from build123d import *

# Parameters (mm, degrees)
F0_W     = 12.1070817113
F0_H     = 12.026887387
F1_DEPTH = 50.8
F2_R     = 5.08
F3_SIZE  = 5.08
F4_T     = -2.54


with BuildPart() as f1:
    # F0 (on Front) → F1 (new body)
    with BuildSketch(Plane.XZ):
        Polygon((-97.7879613638, 32.6970815659), (-97.7879613638, 44.7239689529), (-85.6808796525, 44.7239689529), (-85.6808796525, 56.0660995543), (-101.5132069588, 56.0660995543), (-101.5132069588, 32.6970815659), align=None)
        with Locations((-91.7344205081, 38.7105252594)):
            Rectangle(F0_W, F0_H)
        Polygon((-49.3596345186, 44.7239689529), (-85.6808796525, 44.7239689529), (-85.6808796525, 32.6970815659), (-97.7879613638, 32.6970815659), (-97.7879613638, 15.5531428754), (-49.3596345186, 15.5531428754), align=None)
    extrude(amount=F1_DEPTH)

    # F2
    f2_edges = [f1.edges().sort_by_distance(p)[0] for p in [
        (-85.68088, -25.4, 44.723969),
        (-49.359635, -25.4, 44.723969),
    ]]
    fillet(f2_edges, radius=F2_R)

    # F3
    f3_edges = [f1.edges().sort_by_distance(p)[0] for p in [
        (-49.359635, -25.4, 15.553143),
    ]]
    chamfer(f3_edges, length=F3_SIZE)

    # F4
    f4_openings = [f1.faces().sort_by_distance(p)[0] for p in [
        (-76.801986, -50.8, 32.724788),
    ]]
    offset(amount=F4_T, openings=f4_openings, kind=Kind.INTERSECTION)


solid = f1.part
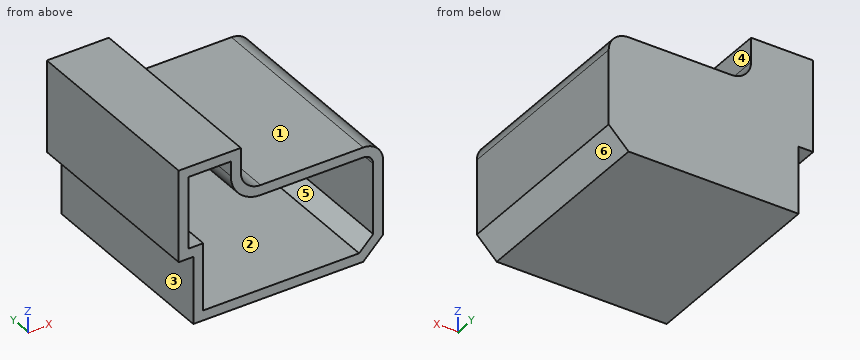
Verification items for the finished model (mm, model axes). Face numbers are marked on the shaded views. A direction names the side the tool comes from. Round coordinates to 2 decimals unless told otherwise and drop trailing zeros. Loops run counter-clockwise (first coordinate to the right, second up) from the corner with the lowest first, then second, coordinate; pieces in that order, holes last. Notation, with made-up numbers: (73, -15.75) - (129, -15.75) arc R25 cw to (129, -0.75) - close; hole circle Ø4 at (54, -10). An arc over 180 degrees is marked (long way). Answer in a Markdown table with one row per item. Add a question column.
Q1. Section check A-A on y = -31. Enter the section's corners in (x, z), plus the area to 3 significant figures.
Q2. Gauge pin test, flat ends, axial feed: pin 1 (2 mm diameter, centred on y = -11, z = 27, fed in from -X); pin 2 (1.9 mm diameter, centred on x = -99, y = -27, fed in from -Z); pin 3 (3 mm diameter, centred on y = -5.5, z = 49, fed in from +X). Record the tip position at first contact, or that the pin passes through.
Q3. Section check C-C on z = 28. Enter the section's corners in (x, y), plus the area to 3 significant figures.
Q4. Tool access check on the marked faces 1, 2 and 3. Record the directions out of +Z, -Z, +X, -X, +Y, -Y that give a thin tool (end or side, any length) a straight path to the whole face; none if there is none.
Q5. Material ranges on line 1 (X direction, y = -26, z = 36); line 2 (Z direction, x = -93, y = -13.5); line 3 (Z direction, x = -72.5, y = -45), recorded low to high.
Q6. Release check for a two-part mould opening along Z. For the marked faces 4, 5 and 6 record: pulls with the +Z half, pulls with the -Z half, needs draft (parallel to the pull), parting line crosses it, or undercut.
Q7. Section check B-B on x = -62.5. Enter the section's corners in (y, z), plus the area to 3 significant figures.
Found:
| question | item | result |
|---|---|---|
| 1 | outline | (-101.51, 32.7) - (-97.79, 32.7) - (-97.79, 15.55) - (-54.44, 15.55) - (-49.36, 20.63) - (-49.36, 39.64) arc R5.08 ccw to (-54.44, 44.72) - (-80.6, 44.72) arc R5.08 cw to (-85.68, 49.8) - (-85.68, 56.07) - (-101.51, 56.07) - close; hole (-98.97, 35.24) - (-95.25, 35.24) - (-95.25, 18.09) - (-55.49, 18.09) - (-51.9, 21.69) - (-51.9, 39.64) arc R2.54 ccw to (-54.44, 42.18) - (-80.6, 42.18) arc R7.62 cw to (-88.22, 49.8) - (-88.22, 53.53) - (-98.97, 53.53) - close |
| 1 | area | 427 mm² |
| 2 | pin 1 | stops at x = -97.79 |
| 2 | pin 2 | stops at z = 32.7 |
| 2 | pin 3 | stops at x = -85.13 |
| 3 | outline | (-97.79, -50.8) - (-95.25, -50.8) - (-95.25, -2.54) - (-51.9, -2.54) - (-51.9, -50.8) - (-49.36, -50.8) - (-49.36, 0) - (-97.79, 0) - close |
| 3 | area | 368 mm² |
| 4 | face 1 | +Z, +X, +Y, -Y |
| 4 | face 2 | -Y |
| 4 | face 3 | -Z, -X, +Y, -Y |
| 5 | line 1 | x = -101.51 to -98.97, -51.9 to -49.36 |
| 5 | line 2 | z = 15.55 to 18.09, 53.53 to 56.07 |
| 5 | line 3 | z = 15.55 to 18.09, 42.18 to 44.72 |
| 6 | face 4 | needs draft |
| 6 | face 5 | undercut |
| 6 | face 6 | pulls with the -Z half |
| 7 | outline | (-50.8, 15.55) - (0, 15.55) - (0, 44.72) - (-50.8, 44.72) - (-50.8, 42.18) - (-2.54, 42.18) - (-2.54, 18.09) - (-50.8, 18.09) - close |
| 7 | area | 319 mm² |
